Check sheet for the modelled part. Datum: model origin and axes. Units: mm. Face numbers are marked on the shaded views. Give positions to 0.01 mm unless a question says otherwise; leave off trailing zeros. Loops run counter-clockwise (first coordinate to the right, second up) from the corner with the lowest first, then second, coordinate; pieces in that order, holes last. Notation, with made-up numbers: M 57.5,-17 L 91.5,-17 A15 cw 91.5,-10 Z; hole C -21,-9 d11. An arc over 180 degrees is marked long. Write each question's results on one line, items separated by ' | '. Start each with the question number.
1. Sectioned sample at B-B on y = 7. Record the cut outline in (x, z).
2. Draft check along Y on the marked faces 1, 2 and 3. Enter one of: pulls with the +Y half, pulls with the -Y half, needs draft (parallel to the pull), parting line crosses it, or undercut.
3. Sectioned sample at D-D on z = -11.5. Record the cut outline in (x, y).
4. Material ranges on line 1 along X through (y, z) = (-13.5, -7); line 2 along Z through (x, y) = (16, 0); line 3 along X through (y, z) = (6, -4.5), recorded low to high.
5. Sectioned sample at C-C on x = -11.5. Record the cut outline in (y, z).
6. Sectioned sample at A-A on x = 0. Record the cut outline in (y, z), and give its area (3 significant figures).
7. Go/stop test with flat-tipped pins: pin 1 (3.5 mm diameter, centred on x = 19, y = 0, fed in from -Z); pin 2 (1.5 mm diameter, centred on y = 2, z = -21.5, fed in from +X); pin 3 (6 mm diameter, centred on y = -2.5, z = -18, fed in from +X); pin 4 (2 mm diameter, centred on x = 17, y = 0, fed in from -Z). Record where each tip stops, or that it passes through.
```python
from build123d import *

# Parameters (mm, degrees)
SKETCH1_R            = 14
SKETCH1_R_2          = 8
BOSS_EXTRUDE1_DEPTH  = 42
SKETCH2_R            = 8
BOSS_EXTRUDE2_DEPTH  = 10
M5_CLEARANCE_HOLE1_D = 5.5


with BuildPart() as part:
    # Sketch1 → Boss-Extrude1 (new body)
    with BuildSketch(Plane.XY):
        Circle(SKETCH1_R)
        Circle(SKETCH1_R_2, mode=Mode.SUBTRACT)
    extrude(amount=-BOSS_EXTRUDE1_DEPTH)

    # Sketch2 → Boss-Extrude2 (add)
    with BuildSketch(Plane.XY):
        with BuildLine():
            Line((13.266499161, 20), (-13.266499161, 20))
            ThreePointArc((-13.266499161, 20), (-24, 0), (-13.266499161, -20))
            Line((-13.266499161, -20), (13.266499161, -20))
            ThreePointArc((13.266499161, -20), (21.147056295, -11.349097324), (24, 0))
            ThreePointArc((24, 0), (21.147056295, 11.349097324), (13.266499161, 20))
        make_face()
        Circle(SKETCH2_R, mode=Mode.SUBTRACT)
    extrude(amount=-BOSS_EXTRUDE2_DEPTH)

    # M5 Clearance Hole1 (through all)
    with Locations(Plane.XY):
        with Locations((-19, 0), (-13.435028843, 13.435028843), (13.435028843, -13.435028843), (0, 0), (13.435028843, 13.435028843), (-13.435028843, -13.435028843), (19, 0)):
            Hole(M5_CLEARANCE_HOLE1_D / 2)


solid = part.part
```
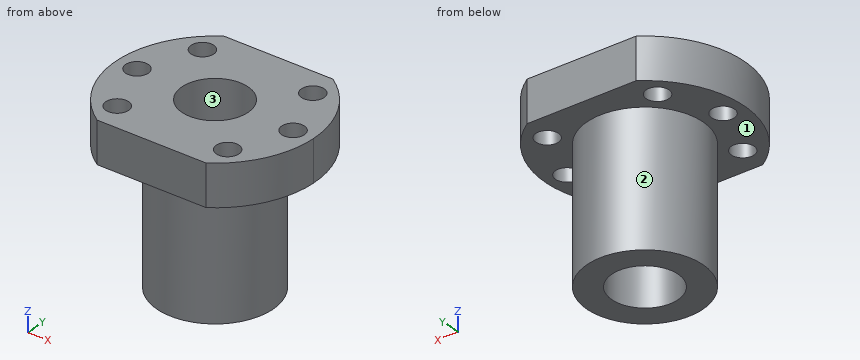
Output values:
1) outline: M -22.96,-10 L -12.12,-10 L -12.12,-42 L -3.87,-42 L -3.87,0 L -22.96,0 Z; M 3.87,-42 L 12.12,-42 L 12.12,-10 L 22.96,-10 L 22.96,0 L 3.87,0 Z
2) face 1: needs draft | face 2: parting line crosses it | face 3: undercut
3) outline: C 0,0 d28; hole C 0,0 d16
4) line 1: -19.84 to -16.18, -10.69 to 10.69, 16.18 to 19.84 | line 2: -10 to 0 | line 3: -23.24 to -5.29, 5.29 to 23.24
5) outline: M -20,-10 L -15.39,-10 L -15.39,0 L -20,0 Z; M -11.48,-10 L -7.98,-10 L -7.98,-42 L 7.98,-42 L 7.98,-10 L 11.48,-10 L 11.48,0 L -11.48,0 Z; M 15.39,-10 L 20,-10 L 20,0 L 15.39,0 Z
6) outline: M -20,-10 L -14,-10 L -14,-42 L -8,-42 L -8,0 L -20,0 Z; M 8,-42 L 14,-42 L 14,-10 L 20,-10 L 20,0 L 8,0 Z | area: 624 mm2
7) pin 1: through | pin 2: x = 13.94 | pin 3: x = 14 | pin 4: z = -10
